```python
from build123d import *

# Parameters (mm, degrees)
CROQUIS1_R                    = 45
SALIENTE_EXTRUIR1_DEPTH       = 6
TALADRO_ROSCADO_M41_D         = 3.3
TALADRO_ROSCADO_M41_DEPTH     = 20
TALADRO_ROSCADO_M41_TIP       = 0.991420021
TALADRO_ROSCADO_M42_D         = 3.3
TALADRO_ROSCADO_M42_DEPTH     = 20
TALADRO_ROSCADO_M42_TIP       = 0.991420021
CORTAR_EXTRUIR1_DEPTH         = 1
CROQUIS7_R                    = 3.25
CORTAR_EXTRUIR2_DEPTH         = 37.7
CROQUIS8_R                    = 5
CORTAR_EXTRUIR3_DEPTH         = 6
TALADRO_ROSCADO_M6X0_51_D     = 5.5
TALADRO_ROSCADO_M6X0_51_DEPTH = 22.5
TALADRO_ROSCADO_M6X0_51_TIP   = 1.652366702
TALADRO_ROSCADO_M6X0_52_D     = 5.5
TALADRO_ROSCADO_M6X0_52_DEPTH = 10.5
TALADRO_ROSCADO_M6X0_52_TIP   = 1.652366702
TALADRO_ROSCADO_M81_D         = 6.8


with BuildPart() as part:
    # Croquis1 → Saliente-Extruir1 (new body, symmetric)
    with BuildSketch(Plane.XY):
        with BuildLine():
            Line((-54.5, 0), (-54.5, 104))
            Line((-54.5, 104), (34.5, 104))
            Line((34.5, 104), (54.5, 94))
            Line((54.5, 94), (54.5, 0))
            ThreePointArc((54.5, 0), (0, -54.5), (-54.5, 0))
        make_face()
        Circle(CROQUIS1_R, mode=Mode.SUBTRACT)
    extrude(amount=SALIENTE_EXTRUIR1_DEPTH, both=True)

    # Taladro roscado M41
    with Locations(Plane(origin=(48.5, 97, 0), x_dir=(-0.894427191, 0.447213595, 0), z_dir=(0.447213595, 0.894427191, 0))):
        with Locations((4.291796068, -1)):
            Hole(TALADRO_ROSCADO_M41_D / 2, depth=TALADRO_ROSCADO_M41_DEPTH)
            with Locations((0, 0, -(TALADRO_ROSCADO_M41_DEPTH + TALADRO_ROSCADO_M41_TIP / 2))):  # 118° drill point
                Cone(0, TALADRO_ROSCADO_M41_D / 2, TALADRO_ROSCADO_M41_TIP, mode=Mode.SUBTRACT)

    # Taladro roscado M42
    with Locations(Plane(origin=(0, 104, 0), x_dir=(-1, 0, 0), z_dir=(0, 1, 0))):
        with Locations((9.5, -1), (-24.9, -1)):
            Hole(TALADRO_ROSCADO_M42_D / 2, depth=TALADRO_ROSCADO_M42_DEPTH)
            with Locations((0, 0, -(TALADRO_ROSCADO_M42_DEPTH + TALADRO_ROSCADO_M42_TIP / 2))):  # 118° drill point
                Cone(0, TALADRO_ROSCADO_M42_D / 2, TALADRO_ROSCADO_M42_TIP, mode=Mode.SUBTRACT)

    # Croquis6 → Cortar-Extruir1 (cut)
    with BuildSketch(Plane.XY.offset(6)):
        with BuildLine():
            Line((40.5, 104), (65.659367038, 104))
            Line((65.659367038, 104), (65.659367038, 19.6))
            Line((65.659367038, 19.6), (45.5, 19.6))
            ThreePointArc((45.5, 19.6), (41.964466094, 21.064466094), (40.5, 24.6))
            Line((40.5, 24.6), (40.5, 104))
        make_face()
    extrude(amount=-CORTAR_EXTRUIR1_DEPTH, mode=Mode.SUBTRACT)

    # Croquis7 → Cortar-Extruir2 (cut)
    with BuildSketch(Plane.XY.offset(5)):
        with Locations((49, 84)):
            Circle(CROQUIS7_R)
        with Locations((49, 34)):
            Circle(CROQUIS7_R)
    extrude(amount=-CORTAR_EXTRUIR2_DEPTH, mode=Mode.SUBTRACT)

    # Croquis8 → Cortar-Extruir3 (cut)
    with BuildSketch(Plane(origin=(0, 0, -6), x_dir=(-1, 0, 0), z_dir=(0, 0, -1))):
        with Locations((-49, 84)):
            Circle(CROQUIS8_R)
        with Locations((-49, 34)):
            Circle(CROQUIS8_R)
    extrude(amount=-CORTAR_EXTRUIR3_DEPTH, mode=Mode.SUBTRACT)

    # Taladro roscado M6x0.51
    with Locations(Plane.ZY.offset(54.5)):
        with Locations((0, 96.5), (0, 51.7)):
            Hole(TALADRO_ROSCADO_M6X0_51_D / 2, depth=TALADRO_ROSCADO_M6X0_51_DEPTH)
            with Locations((0, 0, -(TALADRO_ROSCADO_M6X0_51_DEPTH + TALADRO_ROSCADO_M6X0_51_TIP / 2))):  # 118° drill point
                Cone(0, TALADRO_ROSCADO_M6X0_51_D / 2, TALADRO_ROSCADO_M6X0_51_TIP, mode=Mode.SUBTRACT)

    # Taladro roscado M6x0.52
    with Locations(Plane.ZY.offset(54.5)):
        with Locations((0, 7.5)):
            Hole(TALADRO_ROSCADO_M6X0_52_D / 2, depth=TALADRO_ROSCADO_M6X0_52_DEPTH)
            with Locations((0, 0, -(TALADRO_ROSCADO_M6X0_52_DEPTH + TALADRO_ROSCADO_M6X0_52_TIP / 2))):  # 118° drill point
                Cone(0, TALADRO_ROSCADO_M6X0_52_D / 2, TALADRO_ROSCADO_M6X0_52_TIP, mode=Mode.SUBTRACT)

    # Taladro roscado M81 (through all)
    with Locations(Plane.XY.offset(6)):
        with Locations((0, 63)):
            Hole(TALADRO_ROSCADO_M81_D / 2)


with BuildPart() as body_2:
    # Simetría1: mirrored copy
    add(part.part.mirror(Plane.XY.offset(-6)))


solid = body_2.part
```
For this review, take the finished solid that the model builds, in its own axes (mm). A direction names the side the tool comes from. Give positions to 0.01 mm unless a question says otherwise; leave off trailing zeros. Loops run counter-clockwise (first coordinate to the right, second up) from the corner with the lowest first, then second, coordinate; pieces in that order, holes last. Notation, with made-up numbers: M 48,1 L 100,1 A16 cw 100,25 Z; hole C 44,32.25 d7. An arc over 180 degrees is marked long. One line per item, written item: value. Start each with the question number.
Q1. Clearance check with flat-ended pins moving along their axes: pin 1 Ø0.8 at (y, z) = (69, -17.5) entering from +X; pin 2 Ø0.5 at (x, z) = (48, -17.5) entering from +Y; pin 3 Ø1.5 at (x, z) = (37, -10.5) entering from -Y; pin 4 Ø3 at (x, y) = (48.5, 33.5) entering from +Z. State where each tip first meets the part, or that it passes through.
Q2. For L1, parallel to Y at x = 0, z = -12.25; L2, parallel to X at y = 96, z = -11; L3, parallel to Y at x = -41.5, z = -10.25, list the stretches that pass through material, from the lowest coordinate up.
Q3. Add section D-D (y = 34). Give the boundary of the cut face in (x, z), and give its area (3 significant figures).
Q4. Add section A-A (y = 63). Give the boundary of the cut face in (x, z), and give its area (3 significant figures).
Q5. Draft analysis for pull direction Z (two halves, no side actions). For faces 1 (the face through (0.74, 59.68, -11.92)), 2 (the face through (48, 30.7, -12)), 3 (the face through (-30.635, 52.103, -12.257)), state which applies: released by +Z, released by -Z, zero draft, split by the parting line, or undercut.
Q6. Add section C-C (x = -42). Give the boundary of the cut face in (y, z).
Q7. Machinability: for faces 4 (the face through (-9.9, 93.9, -9.4)), 5 (the face through (42, 21.03, -17.51)), 6 (the face through (45.7, 83, -12)), 7 (the face through (-43.092, 93.815, -12.596)), 8 (the face through (35.106, 80.42, -11.086)), which of the approach directions +Z, -Z, +X, -X, +Y, -Y give a long, thin tool a straight path to every point of the face, cutting with its end or side? Answer none if there is none.
Q8. Add section B-B (x = 0). Give the boundary of the cut face in (y, z), and give its area (3 significant figures).
Reply:
1. pin 1: x = 40.5
1. pin 2: y = 19.6
1. pin 3: y = -40.7
1. pin 4: through
2. L1: -54.5 to -45, 45 to 59.6, 66.4 to 104
2. L2: -31.02 to -11.15, -7.85 to 23.25, 26.55 to 41.36, 45.05 to 50.5
2. L3: -35.33 to -17.4, 17.4 to 49.58, 53.82 to 94.38, 98.62 to 104
3. outline: M -54.5,-18 L -29.48,-18 L -29.48,-6 L -54.5,-6 Z; M 29.48,-18 L 40.5,-18 L 40.5,-17 L 45.75,-17 L 45.75,-12 L 44,-12 L 44,-6 L 29.48,-6 Z; M 52.25,-17 L 54.5,-17 L 54.5,-6 L 54,-6 L 54,-12 L 52.25,-12 Z
3. area: 494 mm²
4. outline: M -54.5,-18 L -3.4,-18 L -3.4,-6 L -54.5,-6 Z; M 3.4,-18 L 40.5,-18 L 40.5,-17 L 54.5,-17 L 54.5,-6 L 3.4,-6 Z
4. area: 1,210 mm²
5. face 1: zero draft
5. face 2: released by +Z
5. face 3: undercut
6. outline: M -34.73,-18 L -16.16,-18 L -16.16,-6 L -34.73,-6 Z; M 16.16,-18 L 104,-18 L 104,-6 L 16.16,-6 Z; hole C 51.7,-12 d5.5; hole C 96.5,-12 d5.5
7. face 4: +Y
7. face 5: -Z, +X, +Y
7. face 6: +Z
7. face 7: -X
7. face 8: none
8. outline: M -54.5,-18 L -45,-18 L -45,-6 L -54.5,-6 Z; M 45,-18 L 59.6,-18 L 59.6,-6 L 45,-6 Z; M 66.4,-18 L 104,-18 L 104,-6 L 66.4,-6 Z
8. area: 740 mm²
